Read the model definition and answer for the solid it produces. Units are mm, in the model's axes. A direction names the side the tool comes from. Give positions to 0.01 mm unless a question says otherwise; leave off trailing zeros. Loops run counter-clockwise (first coordinate to the right, second up) from the corner with the lowest first, then second, coordinate; pieces in that order, holes last. Notation, with made-up numbers: (-7.5, -12.5) - (5.5, -12.5) arc R31 ccw to (5.5, 25.5) - close; hole circle Ø4 at (-1, -29). An arc over 180 degrees is marked (long way). Put each result on its own line as item: value. Start each with the question number.
1. A cutting plane is placed at A-A, the plane y = 12. Determine the outline of the cut face in (x, z), plus the area to 3 significant figures.
2. Given pin 1 Ø12 at (x, y) = (-10.5, -7.5) entering from -Z; pin 2 Ø1.5 at (x, z) = (1.5, 2.5) entering from +Y; pin 3 Ø1.5 at (y, z) = (-4, 0.5) entering from -X; pin 4 Ø2 at (x, z) = (-18, 2.5) entering from -Y, each flat-ended and moving along its own axis, determine where each tip first touches the part or whether it passes through.
3. A cutting plane is placed at B-B, the plane z = 1.15. Determine the outline of the cut face in (x, y).
4. A cutting plane is placed at D-D, the plane y = 8. Determine the outline of the cut face in (x, z), plus the area to 3 significant figures.
5. For a pull along X with two mould halves and no side action, classify faces 1 (the cylindrical face through (-18.19, 13, 2.46)), 2 (the flat face through (0, 1, 0)), 3 (the flat face through (11.03, 9.09, 2.46)), 4 (the flat face through (21.058, -0.588, 2.465)) as released by +X, released by -X, zero draft, split by the parting line, or undercut.
6. A cutting plane is placed at C-C, the plane x = 10.5. Determine the outline of the cut face in (y, z), plus the area to 3 significant figures.
7. Consider L1, parallel to Y at x = -5.5, z = 3.7; L2, parallel to Y at x = 10.5, z = 1.25; L3, parallel to X at y = -9.5, z = 1.3. Determine where each line is inside the solid, lowest interval first. Write a range as from..to.
8. For faces 5 (the flat face through (0, 2.984, 2)), 6 (the cylindrical face through (-16.1, -14, 2.5)), determine the directions among +Z, -Z, +X, -X, +Y, -Y from which every point of the face is accessible in a straight line to the end or side of a thin tool.
```python
from build123d import *

# Parameters (mm, degrees)
SZKIC1_R                    = 1.65
DODANIE_WYCI_GNI_CIE1_DEPTH = 5


with BuildPart() as part:
    # Szkic1 → Dodanie-wyciągnięcie1 (new body)
    with BuildSketch(Plane.XY):
        with BuildLine():
            Line((17.853722756, -11.434054451), (24.353722756, 10.565945549))
            ThreePointArc((24.353722756, 10.565945549), (21.762078084, 16.527487106), (15.438744243, 15.020155366))
            Line((15.438744243, 15.020155366), (6.487805254, 2.983671115))
            Line((6.487805254, 2.983671115), (-6.487805254, 2.983671115))
            Line((-6.487805254, 2.983671115), (-15.438744243, 15.020155366))
            ThreePointArc((-15.438744243, 15.020155366), (-21.762078084, 16.527487106), (-24.353722756, 10.565945549))
            Line((-24.353722756, 10.565945549), (-17.853722756, -11.434054451))
            ThreePointArc((-17.853722756, -11.434054451), (-16.029619333, -14.054200717), (-13, -15.061139867))
            Line((-13, -15.061139867), (13, -15.061139867))
            ThreePointArc((13, -15.061139867), (16.029619333, -14.054200717), (17.853722756, -11.434054451))
        make_face()
        with Locations((10.5, 0)):
            Circle(SZKIC1_R, mode=Mode.SUBTRACT)
        with Locations((19.5, 12)):
            Circle(SZKIC1_R, mode=Mode.SUBTRACT)
        with Locations((13, -10)):
            Circle(SZKIC1_R, mode=Mode.SUBTRACT)
        with Locations(Location((-13, -10, 0), (0, 0, 180))):
            Circle(SZKIC1_R, mode=Mode.SUBTRACT)
        with Locations(Location((-19.5, 12, 0), (0, 0, 180))):
            Circle(SZKIC1_R, mode=Mode.SUBTRACT)
        with Locations(Location((-10.5, 0, 0), (0, 0, 180))):
            Circle(SZKIC1_R, mode=Mode.SUBTRACT)
    extrude(amount=DODANIE_WYCI_GNI_CIE1_DEPTH)


solid = part.part
```
Return value:
1. outline: (-24.56, 0) - (-21.15, 0) - (-21.15, 5) - (-24.56, 5) - close; (-17.85, 0) - (-13.19, 0) - (-13.19, 5) - (-17.85, 5) - close; (13.19, 0) - (17.85, 0) - (17.85, 5) - (13.19, 5) - close; (21.15, 0) - (24.56, 0) - (24.56, 5) - (21.15, 5) - close
1. area: 80.7 mm2
2. pin 1: stops at z = 0
2. pin 2: stops at y = 2.98
2. pin 3: stops at x = -20.27
2. pin 4: stops at y = -13.1
3. outline: (-24.35, 10.57) - (-17.85, -11.43) arc R5.06 ccw to (-13, -15.06) - (13, -15.06) arc R5.06 ccw to (17.85, -11.43) - (24.35, 10.57) arc R5.06 ccw to (15.44, 15.02) - (6.49, 2.98) - (-6.49, 2.98) - (-15.44, 15.02) arc R5.06 ccw to start; hole circle Ø3.3 at (-19.5, 12); hole circle Ø3.3 at (-13, -10); hole circle Ø3.3 at (-10.5, 0); hole circle Ø3.3 at (10.5, 0); hole circle Ø3.3 at (13, -10); hole circle Ø3.3 at (19.5, 12)
4. outline: (-23.6, 0) - (-10.22, 0) - (-10.22, 5) - (-23.6, 5) - close; (10.22, 0) - (23.6, 0) - (23.6, 5) - (10.22, 5) - close
4. area: 134 mm2
5. face 1: undercut
5. face 2: zero draft
5. face 3: undercut
5. face 4: released by +X
6. outline: (-15.06, 0) - (-1.65, 0) - (-1.65, 5) - (-15.06, 5) - close; (1.65, 0) - (8.38, 0) - (8.38, 5) - (1.65, 5) - close
6. area: 101 mm2
7. L1: y = -15.06..2.98
7. L2: y = -15.06..-1.65, 1.65..8.38
7. L3: x = -18.43..-14.57, -11.43..11.43, 14.57..18.43
8. face 5: +Z, -Z, +Y
8. face 6: +Z, -Z, -X, -Y
